Can you work these out from the drawing? Everything is in mm from the part's minimum corner. A direction names the side the tool comes from. Round coordinates to 2 decimals unless told otherwise and drop trailing zeros. Write each loop counter-clockwise with the first axis right and the second up, starting at its lowest first coordinate (ties: lowest second). Pieces come first, ordered by that corner, then holes. Notation, with made-up numbers: M -35.75,-4 L -16.75,-4 A38 cw -16.75,34 Z; hole C 87.5,34.5 d11. An arc over 180 degrees is marked long. Use a Markdown table: item, result. Add a question column.
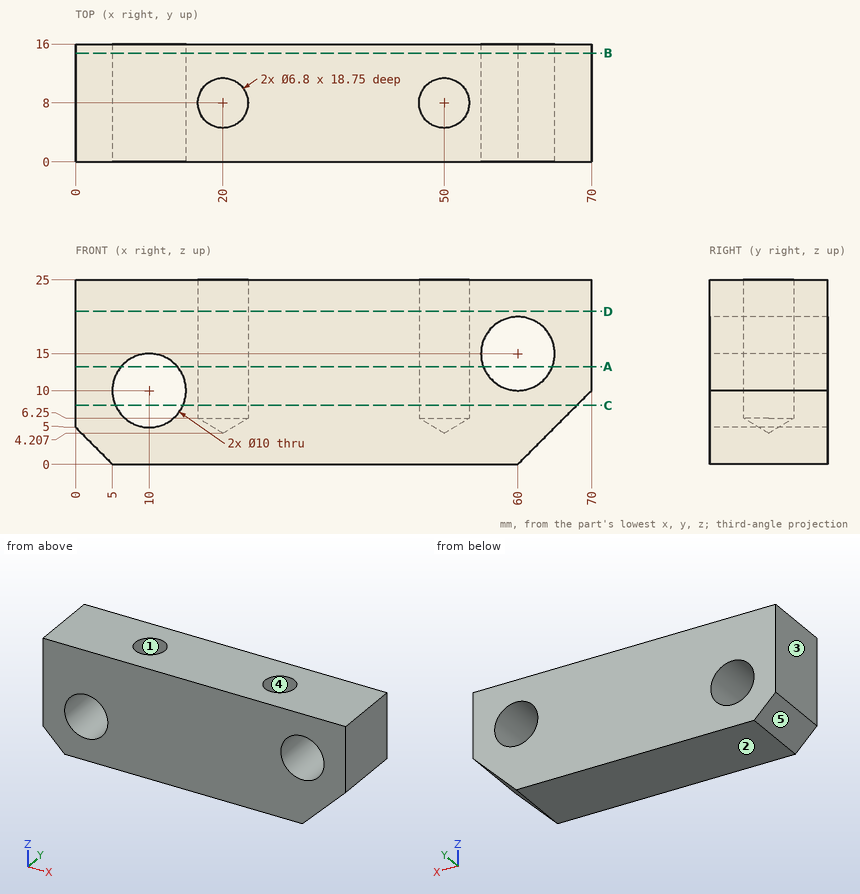
Item 1: Imagine slicing it at C-C on z = 8. List the corners of the cut face in (x, y) for me.
Item 2: On a 3-axis mill with a long thin cutter (end or side, diameter ignored), from which of +Z, -Z, +X, -X, +Y, -Y can I reach the whole of each face in a straight line? I mean the marked faces 4 and 5. Say none if no direction works.
Item 3: Imagine slicing it at D-D on z = 20.75. List the corners of the cut face in (x, y) for me, plus the area to 3 significant figures.
Item 4: Imagine slicing it at B-B on y = 14.75. List the corners of the cut face in (x, z) for me.
Item 5: I need wall thicknesses on probe 1 along Z at (x, y) = (10, 9); probe 2 along Y at (x, z) = (50, 17); probe 3 along Z at (x, y) = (60, 8). Which ranges of each line are inside material? Lowest first, please. Write a range as from..to.
Item 6: For pin 1 Ø8 at (x, z) = (60, 15) entering from -Y; pin 2 Ø3 at (y, z) = (9, 8) entering from +X; pin 3 Ø2 at (x, y) = (48.5, 9) entering from +Z; pin 4 Ø4 at (x, y) = (50, 8) entering from +Z, each with a flat end and sliding along its axis, tell me the tip position at first contact or that it passes through.
Item 7: If we mould it in two halves opening along X, with no side actions, what happens to the marked faces 1, 2 and 3? For each: +X half, -X half, draft (parallel to the pull), parting line (faces both ways), or undercut.
Item 8: Imagine slicing it at A-A on z = 13.25. List the corners of the cut face in (x, y) for me, plus the area to 3 significant figures.
The answers:
| question | item | result |
|---|---|---|
| 1 | outline | M 0,0 L 5.42,0 L 5.42,16 L 0,16 Z; M 14.58,0 L 68,0 L 68,16 L 14.58,16 Z; hole C 20,8 d6.8; hole C 50,8 d6.8 |
| 2 | face 4 | +Z |
| 2 | face 5 | -Z, -X, +Y, -Y |
| 3 | outline | M 0,0 L 70,0 L 70,16 L 0,16 Z; hole C 20,8 d6.8; hole C 50,8 d6.8 |
| 3 | area | 1,050 mm² |
| 4 | outline | M 0,5 L 5,0 L 60,0 L 70,10 L 70,25 L 0,25 Z; hole C 10,10 d10; hole C 60,15 d10 |
| 5 | probe 1 | 0..5, 15..25 |
| 5 | probe 2 | 0..4.6, 11.4..16 |
| 5 | probe 3 | 0..10, 20..25 |
| 6 | pin 1 | through |
| 6 | pin 2 | x = 69.5 |
| 6 | pin 3 | z = 5.89 |
| 6 | pin 4 | z = 5.41 |
| 7 | face 1 | undercut |
| 7 | face 2 | draft |
| 7 | face 3 | -X half |
| 8 | outline | M 0,0 L 6.2,0 L 6.2,16 L 0,16 Z; M 13.8,0 L 55.32,0 L 55.32,16 L 13.8,16 Z; M 64.68,0 L 70,0 L 70,16 L 64.68,16 Z; hole C 20,8 d6.8; hole C 50,8 d6.8 |
| 8 | area | 776 mm² |
